Can you work these out from the model? Positions are in its coordinate system, mm. Face numbers are marked on the shaded views. Give positions to 0.01 mm unless a question says otherwise; leave off trailing zeros. Order: outer loops, then holes, each group sorted by start corner. A loop starts at its lowest first (then second) coordinate and runs counter-clockwise, first axis right, second up.
Item 1: I want a section at D-D, the plane z = 31. Write out the boundary of the cut face in (x, y), then the cut area to 3 significant figures.
Item 2: I want a section at A-A, the plane y = 0. Write out the boundary of the cut face in (x, z), then the cut area to 3 significant figures.
Item 3: If we mould it in two halves opening along Y, with no side actions, what happens to the marked faces 1 and 2? For each: +Y half, -Y half, draft (parallel to the pull), parting line (faces both ways), or undercut.
Item 4: If I drill on line 1 along X through (y, z) = (19.55, -38); line 2 along Y through (x, z) = (-14, -34.5); line 3 along Y through (x, z) = (-9, 17), over which ranges is the centre line in solid material (lowest first)?
Item 5: I want a section at C-C, the plane x = -13.5. Write out the boundary of the cut face in (y, z).
Item 6: I'm going to push flat-ended pins straight in: pin 1 Ø4 at (x, z) = (-13.5, 38) entering from -Y; pin 2 Ø5 at (x, y) = (-8, -9) entering from +Z; pin 3 Ø1 at (x, y) = (13, -4) entering from -Z. Where does each tip first touch, or does it pass through?
Item 7: I want a section at B-B, the plane z = -4.5. Write out the boundary of the cut face in (x, y).
```python
from build123d import *

# Parameters (mm, degrees)
SKETCH1_R                = 15.65
SKETCH1_R_2              = 12.65
BOSS_EXTRUDE1_DEPTH      = 17.5
SKETCH5_R                = 1.6
BOSS_EXTRUDE4_DEPTH      = 2.5
FILLET1_R                = 2
BOSS_EXTRUDE5_REACH      = 57.116
BOSS_EXTRUDE5_END_RADIUS = 15.65
SKETCH6_W                = 13
SKETCH6_H                = 35


with BuildPart() as part:
    # Sketch1 → Boss-Extrude1 (new, symmetric)
    with BuildSketch(Plane.XY):
        Circle(SKETCH1_R)
        Circle(SKETCH1_R_2, mode=Mode.SUBTRACT)
    extrude(amount=BOSS_EXTRUDE1_DEPTH, both=True)



with BuildPart() as body_2:
    # Sketch5 → Boss-Extrude4 (new body)
    # profile 1 of 5: a face of its own
    with BuildSketch(Plane(origin=(0, 20, 0), x_dir=(1, 0, 0), z_dir=(0, 1, 0))):
        with BuildLine():
            Line((-9.576904887, -17.995704843), (-16.272205934, -36.84173742))
            ThreePointArc((-16.272205934, -36.84173742), (-14.449596204, -40.672937463), (-10.618396161, -38.850327734))
            Line((-10.618396161, -38.850327734), (-3.923095113, -20.004295157))
            Line((-3.923095113, -20.004295157), (0, -8.961508912))
            Line((0, -8.961508912), (3.923095113, -20.004295157))
            Line((3.923095113, -20.004295157), (10.618396161, -38.850327734))
            ThreePointArc((10.618396161, -38.850327734), (14.449596204, -40.672937463), (16.272205934, -36.84173742))
            Line((16.272205934, -36.84173742), (9.576904887, -17.995704843))
            Line((9.576904887, -17.995704843), (3.183693955, 0))
            Line((3.183693955, 0), (9.576904887, 17.995704843))
            Line((9.576904887, 17.995704843), (16.272205934, 36.84173742))
            ThreePointArc((16.272205934, 36.84173742), (14.449596204, 40.672937463), (10.618396161, 38.850327734))
            Line((10.618396161, 38.850327734), (3.923095113, 20.004295157))
            Line((3.923095113, 20.004295157), (0, 8.961508912))
            Line((0, 8.961508912), (-3.923095113, 20.004295157))
            Line((-3.923095113, 20.004295157), (-10.618396161, 38.850327734))
            ThreePointArc((-10.618396161, 38.850327734), (-14.449596204, 40.672937463), (-16.272205934, 36.84173742))
            Line((-16.272205934, 36.84173742), (-9.576904887, 17.995704843))
            Line((-9.576904887, 17.995704843), (-3.183693955, 0))
            Line((-3.183693955, 0), (-9.576904887, -17.995704843))
        make_face()
        with Locations(Location((13.5, -38, 0), (0, 0, 270))):
            Circle(SKETCH5_R, mode=Mode.SUBTRACT)
        with Locations(Location((-13.5, -38, 0), (0, 0, 270))):
            Circle(SKETCH5_R, mode=Mode.SUBTRACT)
        with Locations(Location((13.5, 38, 0), (0, 0, 270))):
            Circle(SKETCH5_R, mode=Mode.SUBTRACT)
        with Locations(Location((-13.5, 38, 0), (0, 0, 270))):
            Circle(SKETCH5_R, mode=Mode.SUBTRACT)
    # profile 2 of 5: a face of its own
    with BuildSketch(Plane(origin=(0, 20, 0), x_dir=(1, 0, 0), z_dir=(0, 1, 0))):
        with BuildLine():
            Line((-9.576904887, 17.995704843), (-3.183693955, 0))
            Line((-3.183693955, 0), (-9.576904887, -17.995704843))
            ThreePointArc((-9.576904887, -17.995704843), (-7.526597684, 0), (-9.576904887, 17.995704843))
        make_face()
    # profile 3 of 5: a face of its own
    with BuildSketch(Plane(origin=(0, 20, 0), x_dir=(1, 0, 0), z_dir=(0, 1, 0))):
        with BuildLine():
            ThreePointArc((9.576904887, 17.995704843), (7.526597684, 0), (9.576904887, -17.995704843))
            Line((9.576904887, -17.995704843), (3.183693955, 0))
            Line((3.183693955, 0), (9.576904887, 17.995704843))
        make_face()
    # profile 4 of 5: a face of its own
    with BuildSketch(Plane(origin=(0, 20, 0), x_dir=(1, 0, 0), z_dir=(0, 1, 0))):
        with BuildLine():
            Line((-3.923095113, -20.004295157), (0, -8.961508912))
            Line((0, -8.961508912), (3.923095113, -20.004295157))
            ThreePointArc((3.923095113, -20.004295157), (0, -18.380084852), (-3.923095113, -20.004295157))
        make_face()
    # profile 5 of 5: a face of its own
    with BuildSketch(Plane(origin=(0, 20, 0), x_dir=(1, 0, 0), z_dir=(0, 1, 0))):
        with BuildLine():
            ThreePointArc((-3.923095113, 20.004295157), (0, 18.380084852), (3.923095113, 20.004295157))
            Line((3.923095113, 20.004295157), (0, 8.961508912))
            Line((0, 8.961508912), (-3.923095113, 20.004295157))
        make_face()
    extrude(amount=-BOSS_EXTRUDE4_DEPTH)

    # Fillet1
    fillet1_edges = [body_2.edges().sort_by_distance(p)[0] for p in [
        (-9.576904887, 18.75, -17.995704843),
        (-3.923095113, 18.75, -20.004295157),
        (3.923095113, 18.75, -20.004295157),
        (9.576904887, 18.75, -17.995704843),
        (9.576904887, 18.75, 17.995704843),
        (3.923095113, 18.75, 20.004295157),
        (-3.923095113, 18.75, 20.004295157),
        (-9.576904887, 18.75, 17.995704843),
    ]]
    fillet(fillet1_edges, radius=FILLET1_R)


with BuildPart() as part_1:
    add(part.part)

    add(body_2.part)  # Boss-Extrude5 merges body 2
    # Boss-Extrude5: up to this cylinder (the profile starts outside it)
    boss_extrude5_end = Plane(origin=(0, 0, 0), z_dir=(0, 0, -1)) * Cylinder(BOSS_EXTRUDE5_END_RADIUS, 146.532, mode=Mode.PRIVATE)
    # Sketch6 → Boss-Extrude5 (add, up to the surface)
    with BuildSketch(Plane.XZ.offset(-17.5), mode=Mode.PRIVATE) as boss_extrude5_sk1:
        Rectangle(SKETCH6_W, SKETCH6_H)
    boss_extrude5_tool1 = extrude(boss_extrude5_sk1.sketch, amount=BOSS_EXTRUDE5_REACH, mode=Mode.PRIVATE) - boss_extrude5_end
    add(boss_extrude5_tool1.solids().sort_by_distance((0, 17.5, 0))[0])


solid = part_1.part
```
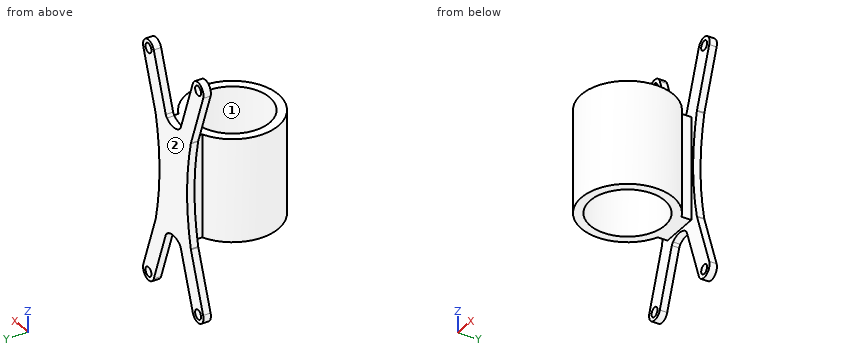
Results list:
1. outline: (-14.2, 17.5) - (-7.83, 17.5) - (-7.83, 20) - (-14.2, 20) - close; (7.83, 17.5) - (14.2, 17.5) - (14.2, 20) - (7.83, 20) - close
1. area: 31.8 mm2
2. outline: (-15.65, -17.5) - (-12.65, -17.5) - (-12.65, 17.5) - (-15.65, 17.5) - close; (12.65, -17.5) - (15.65, -17.5) - (15.65, 17.5) - (12.65, 17.5) - close
2. area: 210 mm2
3. face 1: undercut
3. face 2: +Y half
4. line 1: x = -16.44 to -15.1, -11.9 to -10.32, 10.32 to 11.9, 15.1 to 16.44
4. line 2: y = 17.5 to 20
4. line 3: y = -12.8 to -8.89, 8.89 to 12.8, 17.5 to 20
5. outline: (-7.92, -17.5) - (7.92, -17.5) - (7.92, 17.5) - (-7.92, 17.5) - close; (17.5, -40.85) - (20, -40.85) - (20, -39.6) - (17.5, -39.6) - close; (17.5, -36.4) - (20, -36.4) - (20, -29.04) - (17.5, -29.04) - close; (17.5, 29.04) - (20, 29.04) - (20, 36.4) - (17.5, 36.4) - close; (17.5, 39.6) - (20, 39.6) - (20, 40.85) - (17.5, 40.85) - close
6. pin 1: stops at y = 17.5
6. pin 2: stops at z = 17.5
6. pin 3: stops at z = -17.5
7. outline: (-7.65, 17.5) - (-6.5, 17.5) - (-6.5, 14.24) arc R15.65 ccw (long way) to (6.5, 14.24) - (6.5, 17.5) - (7.65, 17.5) - (7.65, 20) - (-7.65, 20) - close; hole circle Ø25.3 at (0, 0)
